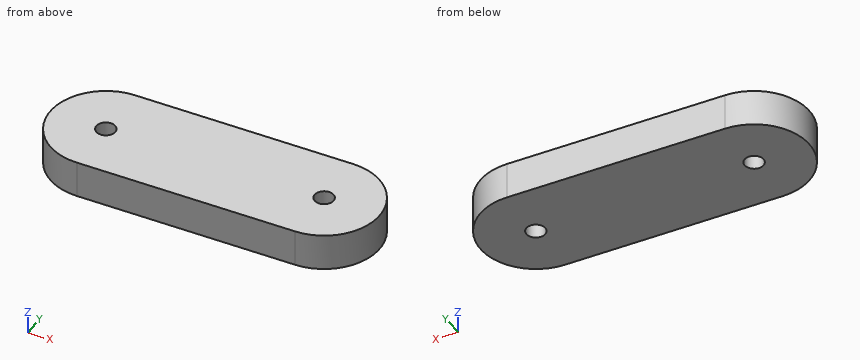
from build123d import *

# Parameters (mm, degrees)
BOSS_EXTRUDE1_DEPTH            = 2
TAP_DRILL_FOR_M2_5X0_45_TAP1_D = 2.05


with BuildPart() as part:
    # Sketch1 → Boss-Extrude1 (new, symmetric)
    with BuildSketch(Plane.XY):
        with BuildLine():
            Line((-11.817810242, 6.443484678), (11.682189758, 6.443484678))
            ThreePointArc((11.682189758, 6.443484678), (17.682189758, 0.443484678), (11.682189758, -5.556515322))
            Line((11.682189758, -5.556515322), (-11.817810242, -5.556515322))
            ThreePointArc((-11.817810242, -5.556515322), (-17.817810242, 0.443484678), (-11.817810242, 6.443484678))
        make_face()
    extrude(amount=BOSS_EXTRUDE1_DEPTH, both=True)

    # Tap Drill for M2.5x0.45 Tap1 (through all)
    with Locations(Plane(origin=(-11.817810242, 0.443484678, 2), x_dir=(1, 0, 0), z_dir=(0, 0, 1))):
        with Locations((0, 0), (23.5, 0)):
            Hole(TAP_DRILL_FOR_M2_5X0_45_TAP1_D / 2)


solid = part.part
Build history of the part. All positions in model axes, mm. Round coordinates to 2 decimals unless told otherwise and drop trailing zeros. Write each loop counter-clockwise with the first axis right and the second up, starting at its lowest first coordinate (ties: lowest second). Pieces come first, ordered by that corner, then holes. Notation, with made-up numbers: M 82.5,-40 L 100.5,-40 A21 cw 100.5,-16 Z; hole C 3.25,31 d5. An arc over 180 degrees is marked long. Answer as a JSON object with one key per item and string values. Group by question number.
(1) Cut at A-A (z = 0.7). Give the cut face in (x, y) (3 decimals).
(2) Cut at B-B (y = -0.25). Give the cut face in (x, z), and give its area (3 significant figures).
(3) Drill centre lines: L1, parallel to X at y = 1, z = 1.3; L2, parallel to Y at x = -12.5, z = 1.5; L3, parallel to Y at x = 12, z = -0.2. Where is each one in solid material? Low to high.
(4) Cut at C-C (x = -15). Give the cut face in (y, z), and give its area (3 significant figures).
(5) Flat gauge pins, fed straight in: pin 1 (1.2 mm diameter, centred on x = 11.68, y = 0.44, fed in from -Z); pin 2 (2 mm diameter, centred on y = -4.5, z = -1, fed in from +X). Where does each tip first touch, or does it go through?
(6) Cut at D-D (y = 3.75). Give the cut face in (x, z), and give its area (3 significant figures).
Responses:
{
 "1": {"outline": "M -11.818,-5.557 L 11.682,-5.557 A6 ccw 11.682,6.443 L -11.818,6.443 A6 ccw Z; hole C -11.818,0.443 d2.05; hole C 11.682,0.443 d2.05"},
 "2": {"outline": "M -17.78,-2 L -12.57,-2 L -12.57,2 L -17.78,2 Z; M -11.06,-2 L 10.93,-2 L 10.93,2 L -11.06,2 Z; M 12.44,-2 L 17.64,-2 L 17.64,2 L 12.44,2 Z", "area": "130 mm2"},
 "3": {"L1": "x = -17.79 to -12.68, -10.96 to 10.82, 12.54 to 17.66", "L2": "y = -5.52 to -0.32, 1.21 to 6.4", "L3": "y = -5.55 to -0.53, 1.42 to 6.44"},
 "4": {"outline": "M -4.64,-2 L 5.53,-2 L 5.53,2 L -4.64,2 Z", "area": "40.7 mm2"},
 "5": {"pin 1": "passes through", "pin 2": "stops at x = 16.2"},
 "6": {"outline": "M -16.82,-2 L 16.69,-2 L 16.69,2 L -16.82,2 Z", "area": "134 mm2"}
}
